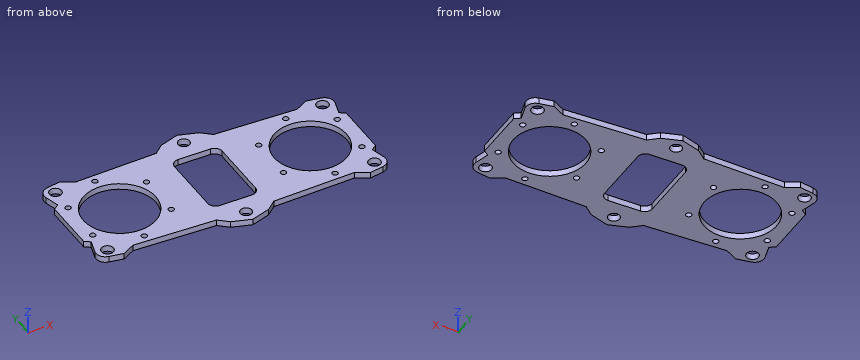
from build123d import *

# Parameters (mm, degrees)
SKETCH1_R           = 3
SKETCH1_R_2         = 19
BOSS_EXTRUDE1_DEPTH = 3.175
CUT_EXTRUDE1_DEPTH  = 4.175
SKETCH3_R           = 3.15
BOSS_EXTRUDE2_DEPTH = 3.175
FILLET1_R           = 5
SKETCH4_R           = 1.5
CUT_EXTRUDE2_DEPTH  = 4.175


with BuildPart() as part:
    # Sketch1 → Boss-Extrude1 (new body)
    with BuildSketch(Plane.XY):
        Polygon((0, 36.5), (-10, 33.28960264), (-15, 29), (-58.05, 27.5), (-76.5, 14), (-76.5, -14), (-58.05, -27.5), (-15, -29), (-10, -33.28960264), (0, -36.5), (10, -33.28960264), (15, -29), (58.05, -27.5), (76.5, -14), (76.5, 14), (58.05, 27.5), (15, 29), (10, 33.28960264), align=None)
        with Locations((0, 30)):
            Circle(SKETCH1_R, mode=Mode.SUBTRACT)
        with Locations((-50, 0)):
            Circle(SKETCH1_R_2, mode=Mode.SUBTRACT)
        with Locations((50, 0)):
            Circle(SKETCH1_R_2, mode=Mode.SUBTRACT)
        with Locations((0, -30)):
            Circle(SKETCH1_R, mode=Mode.SUBTRACT)
    extrude(amount=BOSS_EXTRUDE1_DEPTH)

    # Sketch2 → Cut-Extrude1 (cut, through all)
    with BuildSketch(Plane.XY.offset(3.175)):
        with BuildLine():
            Line((8.5, 20), (-8.5, 20))
            ThreePointArc((-8.5, 20), (-11.328427125, 18.828427125), (-12.5, 16))
            Line((-12.5, 16), (-12.5, -16))
            ThreePointArc((-12.5, -16), (-11.328427125, -18.828427125), (-8.5, -20))
            Line((-8.5, -20), (8.5, -20))
            ThreePointArc((8.5, -20), (11.328427125, -18.828427125), (12.5, -16))
            Line((12.5, -16), (12.5, 16))
            ThreePointArc((12.5, 16), (11.328427125, 18.828427125), (8.5, 20))
        make_face()
    extrude(amount=-CUT_EXTRUDE1_DEPTH, mode=Mode.SUBTRACT)

    # Sketch3 → Boss-Extrude2 (add)
    with BuildSketch(Plane.XY.offset(3.175)):
        Polygon((-58.05, 27.5), (-64.551915182, 31.10998542), (-77.245081729, 28.773819798), (-73.669390597, 16.071177612), align=None)
        with Locations((-70, 25)):
            Circle(SKETCH3_R, mode=Mode.SUBTRACT)
        Polygon((73.669390597, 16.071177612), (58.05, 27.5), (64.551915182, 31.10998542), (77.245081729, 28.773819798), align=None)
        with Locations((70, 25)):
            Circle(SKETCH3_R, mode=Mode.SUBTRACT)
        Polygon((58.05, -27.5), (64.551915182, -31.10998542), (77.245081729, -28.773819798), (73.669390597, -16.071177612), align=None)
        with Locations((70, -25)):
            Circle(SKETCH3_R, mode=Mode.SUBTRACT)
        Polygon((-73.669390597, -16.071177612), (-58.05, -27.5), (-64.551915182, -31.10998542), (-77.245081729, -28.773819798), align=None)
        with Locations((-70, -25)):
            Circle(SKETCH3_R, mode=Mode.SUBTRACT)
    extrude(amount=-BOSS_EXTRUDE2_DEPTH)

    # Fillet1
    fillet1_edges = [part.edges().sort_by_distance(p)[0] for p in [
        (77.245081729, 28.773819798, 1.5875),
        (77.245081729, -28.773819798, 1.5875),
        (-77.245081729, -28.773819798, 1.5875),
        (-77.245081729, 28.773819798, 1.5875),
    ]]
    fillet(fillet1_edges, radius=FILLET1_R)

    # Sketch4 → Cut-Extrude2 (cut, through all)
    with BuildSketch(Plane.XY.offset(3.175)):
        with Locations((-50, 23.75)):
            Circle(SKETCH4_R)
        with Locations((-70.56810334, 11.875)):
            Circle(SKETCH4_R)
        with Locations((-70.56810334, -11.875)):
            Circle(SKETCH4_R)
        with Locations((-50, -23.75)):
            Circle(SKETCH4_R)
        with Locations((-29.43189666, -11.875)):
            Circle(SKETCH4_R)
        with Locations((-29.43189666, 11.875)):
            Circle(SKETCH4_R)
        with Locations((29.43189666, 11.875)):
            Circle(SKETCH4_R)
        with Locations((29.43189666, -11.875)):
            Circle(SKETCH4_R)
        with Locations((50, -23.75)):
            Circle(SKETCH4_R)
        with Locations((70.56810334, -11.875)):
            Circle(SKETCH4_R)
        with Locations((70.56810334, 11.875)):
            Circle(SKETCH4_R)
        with Locations((50, 23.75)):
            Circle(SKETCH4_R)
    extrude(amount=-CUT_EXTRUDE2_DEPTH, mode=Mode.SUBTRACT)


solid = part.part
Input: part model. Units: mm. Frame: model coordinates. Give positions to 0.01 mm unless a question says otherwise; leave off trailing zeros. Loops run counter-clockwise (first coordinate to the right, second up) from the corner with the lowest first, then second, coordinate; pieces in that order, holes last. Notation, with made-up numbers: (22, 49.25) - (27, 49.25) arc R17 ccw to (27, 59.25) - close; hole circle Ø8 at (84, -29.5). An arc over 180 degrees is marked (long way). Use CSV: the item, a comma, the result in double quotes. Start each with the question number.
Item 1: Contact query for flat-ended pins moving along their axis: P1, Ø23, axis at x = 50, y = 0, coming from the +Z side; P2, Ø1.6, axis at x = -1.5, z = 2, coming from the +Y side. Output: stop coordinate, or through.
Item 2: Section D-D on z = 0.5. State how many separate pieces and enclosed holes the cut face has, then the cut area to 3 significant figures.
Item 3: Line query: line 1 (Y direction, x = -50, z = 1.3); line 2 (X direction, y = 0.5, z = 0.55); line 3 (X direction, y = 4.5, z = 2.1). Output: solid intervals per line, ascending.
Item 4: Section C-C on x = 33. Return loops of the section in (y, z) (3 decimals), then the cut area to 3 significant figures.
Item 5: Section A-A on x = 50. Return loops of the section in (y, z) (3 decimals).
Item 6: Section B-B on y = -3. Return loops of the section in (x, z) (3 decimals).
Ans:
1,P1,"passes through"
1,P2,"stops at y = 36.28"
2,separate pieces,"1"
2,enclosed holes,"21"
2,area,"5,470 mm2"
3,line 1,"y = -27.78 to -25.25, -22.25 to -19, 19 to 22.25, 25.25 to 27.78"
3,line 2,"x = -76.5 to -68.99, -31.01 to -12.5, 12.5 to 31.01, 68.99 to 76.5"
3,line 3,"x = -76.5 to -68.46, -31.54 to -12.5, 12.5 to 31.54, 68.46 to 76.5"
4,outline,"(-28.373, 0) - (-8.485, 0) - (-8.485, 3.175) - (-28.373, 3.175) - close; (8.485, 0) - (28.373, 0) - (28.373, 3.175) - (8.485, 3.175) - close"
4,area,"126 mm2"
5,outline,"(-27.78, 0) - (-25.25, 0) - (-25.25, 3.175) - (-27.78, 3.175) - close; (-22.25, 0) - (-19, 0) - (-19, 3.175) - (-22.25, 3.175) - close; (19, 0) - (22.25, 0) - (22.25, 3.175) - (19, 3.175) - close; (25.25, 0) - (27.78, 0) - (27.78, 3.175) - (25.25, 3.175) - close"
6,outline,"(-76.5, 0) - (-68.762, 0) - (-68.762, 3.175) - (-76.5, 3.175) - close; (-31.238, 0) - (-12.5, 0) - (-12.5, 3.175) - (-31.238, 3.175) - close; (12.5, 0) - (31.238, 0) - (31.238, 3.175) - (12.5, 3.175) - close; (68.762, 0) - (76.5, 0) - (76.5, 3.175) - (68.762, 3.175) - close"
